Autodesk Inventor part; units mm, degrees
ref_plane "YZ Plane" through (0, 0, 0) normal (1, 0, 0) x (0, 1, 0)
ref_plane "XZ Plane" through (0, 0, 0) normal (0, 1, 0) x (-1, 0, 0)
ref_plane "XY Plane" through (0, 0, 0) normal (0, 0, 1) x (1, 0, 0)
sketch "Sketch1" plane through (0, 0, 0) normal (0, 0, 1) x (1, 0, 0)
  line L0 (5.475, -45) -> (15, -45)
  line L1 (15, -45) -> (15, 45)
  line L2 (15, 45) -> (5.475, 45)
  line L3 (5.475, -45) -> (15, 45) construction
  line L4 (15, -45) -> (5.475, 45) construction
  arc A0 (0, 15) -> (5.475, 20.475) centre (0, 20.475) ccw
  line L5 (5.475, 0) -> (15, 0) construction
  arc A1 (5.475, -20.475) -> (0, -15) centre (0, -20.475) ccw
  line L6 (5.475, 45) -> (5.475, 20.475)
  line L7 (5.475, -20.475) -> (5.475, -45)
  arc A2 (0, 15) -> (0, -15) centre (0, 0) ccw
  point P0 (10.2375, 0)
  point P1 (10.2375, 0)
  dimension "d1" = 90
  dimension "d2" = 9.525
  dimension "d3" = 15
extrude "Extrusion1" add sketch "Sketch1" along normal blind 30
sketch "Sketch2" plane through (5.475, 20.475, 0) normal (-1, 0, 0) x (0, 0, 1)
  line L0 (0, -65.475) -> (30, -65.475)
  line L1 (0, 24.525) -> (30, 24.525)
  point P0 (0, -20.475)
  point P1 (15, 9.525)
  point P2 (15, -50.475)
  point P3 (15, -65.475)
  dimension "d6" = 15
  dimension "d7" = 15
hole "Hole1" at (5.475, 30, 15) at (5.475, -30, 15) direction (1, 0, 0) diameter 6.604 end through all counterbore diameter 18.0086 counterbore depth 4.8006
fillet "Fillet1" radius 6.35 4 edges at (10.2375, -45, 30) (10.2375, 45, 30) (10.2375, 45, 0) (10.2375, -45, 0)
properties part number "NASA-20-ARM-BR-01"
Can you work these out from the model? Positions are in its coordinate system, mm. A direction names the side the tool comes from. Coordinates: 2 decimals unless noted, no trailing zeros. Write each loop counter-clockwise with the first axis right and the second up, starting at its lowest first coordinate (ties: lowest second). Pieces come first, ordered by that corner, then holes. Notation, with made-up numbers: M 42.25,-8 L 50.25,-8 A4 ccw 50.25,-1 Z; hole C 63.5,14.5 d6. An arc over 180 degrees is marked long. Answer as CSV lines item,"result".
Item 1: Imagine slicing it at B-B on z = 15. List the corners of the cut face in (x, y) for me (3 decimals).
Geometry results:
outline,"M 0,-15 A5.475 cw 5.475,-20.475 L 5.475,-20.996 L 10.276,-20.996 L 10.276,-26.698 L 15,-26.698 L 15,26.698 L 10.276,26.698 L 10.276,20.996 L 5.475,20.996 L 5.475,20.475 A5.475 cw 0,15 A15 ccw Z; M 5.475,-45 L 15,-45 L 15,-33.302 L 10.276,-33.302 L 10.276,-39.004 L 5.475,-39.004 Z; M 5.475,39.004 L 10.276,39.004 L 10.276,33.302 L 15,33.302 L 15,45 L 5.475,45 Z"
Item 2: Please list where these lines run through material, in increasing order: line 1 along Y through (x, z) = (12.75, 15); line 2 along Y through (x, z) = (8.35, 15); line 3 along Z through (x, y) = (8.4, -30).
Geometry results:
line 1,"y = -45 to -33.3, -26.7 to 26.7, 33.3 to 45"
line 2,"y = -45 to -39, -21 to 21, 39 to 45"
line 3,"z = 0 to 6, 24 to 30"
Item 3: Imagine slicing it at D-D on z = 28. List the corners of the cut face in (x, y) for me (3 decimals).
Geometry results:
outline,"M 0,-15 A5.475 cw 5.475,-20.475 L 5.475,-43.276 L 15,-43.276 L 15,43.276 L 5.475,43.276 L 5.475,20.475 A5.475 cw 0,15 A15 ccw Z"
Item 4: I'm going to push flat-ended pins straight in: P1, Ø4, axis at y = -10, z = 20, coming from the -X side; P2, Ø14.5, axis at y = 27.5, z = 19, coming from the -X side; P3, Ø7.5, axis at y = 30, z = 15, coming from the -X side. Where does each tip first touch, or does it pass through?
Geometry results:
P1,"stops at x = -12.69"
P2,"stops at x = 5.47"
P3,"stops at x = 10.28"
Item 5: We'd pull the mould along Z, two halves only. Please class faces 4 (the cylindrical face through (10.3, -43.19, 1.91)), 5 (the cylindrical face through (12.671, 33.223, 14.284)), 6 (the flat face through (10, -45, 15)): +Z half, -Z half, draft (parallel to the pull), parting line (faces both ways), or undercut.
Geometry results:
face 4,"-Z half"
face 5,"undercut"
face 6,"draft"
Item 6: Imagine slicing it at A-A on y = 30. List the corners of the cut face in (x, z) for me (3 decimals), plus the area to 3 significant figures.
Geometry results:
outline,"M 5.475,0 L 15,0 L 15,11.698 L 10.276,11.698 L 10.276,5.996 L 5.475,5.996 Z; M 5.475,24.004 L 10.276,24.004 L 10.276,18.302 L 15,18.302 L 15,30 L 5.475,30 Z"
area,"168 mm2"
Item 7: On a 3-axis mill with a long thin cutter (end or side, diameter ignored), from which of +Z, -Z, +X, -X, +Y, -Y can I reach the whole of each face in a straight line? I mean faces 1 (the flat face through (10, 45, 15)), 2 (the flat face through (5.475, 41, 15)), 3 (the flat face through (10.276, 30, 19)). Say none if no direction works.
Geometry results:
face 1,"+Z, -Z, +X, -X, +Y"
face 2,"+Z, -Z, -X, +Y"
face 3,"-X"
Item 8: Imagine slicing it at C-C on x = 7.25. List the corners of the cut face in (y, z) for me, plus the area to 3 significant figures.
Geometry results:
outline,"M -45,6.35 A6.35 ccw -38.65,0 L 38.65,0 A6.35 ccw 45,6.35 L 45,23.65 A6.35 ccw 38.65,30 L -38.65,30 A6.35 ccw -45,23.65 Z; hole C -30,15 d18.01; hole C 30,15 d18.01"
area,"2,160 mm2"
